```python
from build123d import *

# Parameters (mm, degrees)
IZIM12_R                = 1.6
KES_EKSTR_ZYON1_DEPTH   = 122.918005233
DAIRESEL_KAPLAMA1_COUNT = 6
KES_EKSTR_ZYON2_START   = 27
IZIM13_R                = 1.25
KES_EKSTR_ZYON2_DEPTH   = 10
DAIRESEL_KAPLAMA2_COUNT = 4


with BuildPart() as part:
    # Çizim1 → Döndür1 (revolve)
    with BuildSketch(Plane.XY, mode=Mode.PRIVATE) as d_nd_r1_sk:
        Polygon((-60, 40), (-60, 37), (-70, 37), (-70, 22), (-108, 22), (-108, 4), (-106, 4), (-106, 18.2), (-57, 18.2), (-57, 32), (0, 32), (0, 36), (-17, 36), (-17, 35), (-20, 35), (-20, 40), align=None)
    revolve(d_nd_r1_sk.sketch.rotate(Axis((-88.99, 0, 0), (1, 0, 0)), 90), axis=Axis((-88.99, 0, 0), (1, 0, 0)))

    # Çizim12 → Kes-Ekstrüzyon1 (cut, through all)
    with BuildSketch(Plane(origin=(0, 0, 0), x_dir=(0, 0, -1), z_dir=(1, 0, 0))):
        with Locations((12.5, 0)):
            Circle(IZIM12_R)
    kes_ekstr_zyon1 = extrude(amount=-KES_EKSTR_ZYON1_DEPTH, mode=Mode.SUBTRACT)

    # Dairesel Kaplama1: Kes-Ekstrüzyon1 ×6 about axis
    dairesel_kaplama1_axis = Axis((0, 0, 0), (1, 0, 0))
    for i in range(1, DAIRESEL_KAPLAMA1_COUNT):
        add(kes_ekstr_zyon1.rotate(dairesel_kaplama1_axis, i * 360 / DAIRESEL_KAPLAMA1_COUNT), mode=Mode.SUBTRACT)

    # Çizim13 → Kes-Ekstrüzyon2 (cut)
    with BuildSketch(Plane.XY.offset(KES_EKSTR_ZYON2_START)):
        with Locations((-65, 0)):
            Circle(IZIM13_R)
    kes_ekstr_zyon2 = extrude(amount=KES_EKSTR_ZYON2_DEPTH, mode=Mode.SUBTRACT)

    # Dairesel Kaplama2: Kes-Ekstrüzyon2 ×4 about axis
    dairesel_kaplama2_axis = Axis((0, 0, 0), (1, 0, 0))
    for i in range(1, DAIRESEL_KAPLAMA2_COUNT):
        add(kes_ekstr_zyon2.rotate(dairesel_kaplama2_axis, i * 360 / DAIRESEL_KAPLAMA2_COUNT), mode=Mode.SUBTRACT)


solid = part.part
```
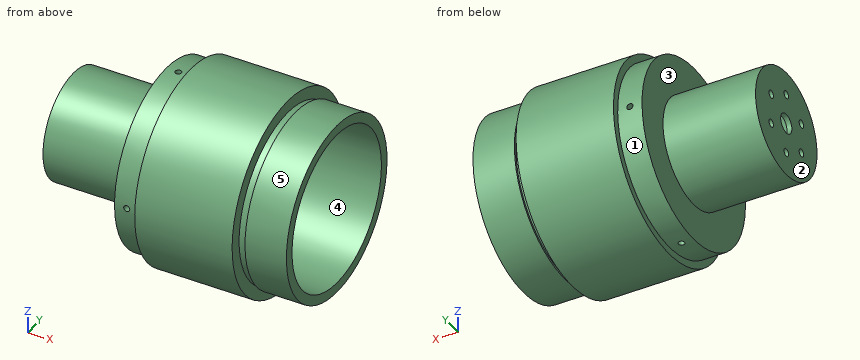
Build history of the part. All positions in model axes, mm. Face numbers are marked on the shaded views. A direction names the side the tool comes from. Round coordinates to 2 decimals unless told otherwise and drop trailing zeros. Write each loop counter-clockwise with the first axis right and the second up, starting at its lowest first coordinate (ties: lowest second). Pieces come first, ordered by that corner, then holes. Notation, with made-up numbers: (28, 18.25) -> (67, 18.25) arc R15 ccw to (67, 23.25) -> close; hole circle Ø3 at (32, 54.5). An arc over 180 degrees is marked (long way). Put each result on its own line as item: value.
Item 1: Wall check: probe 1 along X at (y, z) = (0, -31); probe 2 along Y at (x, z) = (-106.5, 0); probe 3 along X at (y, z) = (21.5, -10). Give the ranges that are in metal, low to high. Write a range as from..to.
Here are the results:
probe 1: x = -70..-66.25, -63.75..-57
probe 2: y = -22..-4, 4..22
probe 3: x = -70..-57
Item 2: Two-plate mould, pull along Z, no slides. Class the marked faces 3, 4 and 5: pulls with the +Z half, pulls with the -Z half, needs draft (parallel to the pull), parting line crosses it, or undercut.
Here are the results:
face 3: needs draft
face 4: undercut
face 5: parting line crosses it
Item 3: Slice it at C-C, the plane z = 30. Give the cut face in (x, y), plus the area to 3 significant figures.
Here are the results:
outline: (-70, -21.66) -> (-60, -21.66) -> (-60, -26.46) -> (-20, -26.46) -> (-20, -18.03) -> (-17, -18.03) -> (-17, -19.9) -> (0, -19.9) -> (0, -11.14) -> (-57, -11.14) -> (-57, 11.14) -> (0, 11.14) -> (0, 19.9) -> (-17, 19.9) -> (-17, 18.03) -> (-20, 18.03) -> (-20, 26.46) -> (-60, 26.46) -> (-60, 21.66) -> (-70, 21.66) -> close; hole circle Ø2.5 at (-65, 0)
area: 2,060 mm^2
Item 4: Flat gauge pins, fed straight in: P1, Ø3, axis at x = -65, z = 0, coming from the -Y side; P2, Ø5, axis at x = -81.5, z = 0, coming from the -Y side; P3, Ø1.5, axis at x = -57.5, z = 24, coming from the +Y side; P4, Ø2.5, axis at y = 10.83, z = 6.25, coming from the +X side. Where does each tip first touch, or does it go through?
Here are the results:
P1: stops at y = -37
P2: stops at y = -22
P3: stops at y = 32.55
P4: passes through
Item 5: Tool access for the marked faces 1 and 2: list every direction of +Z, -Z, +X, -X, +Y, -Y with a clear straight run to the whole face (end or side of a thin tool).
Here are the results:
face 1: -X
face 2: +Z, -Z, -X, +Y, -Y
Item 6: Slice it at B-B, the plane x = -97. Give the cut face in (y, z).
Here are the results:
outline: circle Ø44 at (0, 0); hole circle Ø36.4 at (0, 0)
Item 7: Slice it at D-D, the plane y = 24. Give the cut face in (x, z), plus the area to 3 significant figures.
Here are the results:
outline: (-70, -28.16) -> (-60, -28.16) -> (-60, -32) -> (-20, -32) -> (-20, -25.48) -> (-17, -25.48) -> (-17, -26.83) -> (0, -26.83) -> (0, -21.17) -> (-57, -21.17) -> (-57, 21.17) -> (0, 21.17) -> (0, 26.83) -> (-17, 26.83) -> (-17, 25.48) -> (-20, 25.48) -> (-20, 32) -> (-60, 32) -> (-60, 28.16) -> (-70, 28.16) -> close
area: 1,780 mm^2
